Work out the finished part from the listing and answer in its coordinate system (mm). A direction names the side the tool comes from. Coordinates: 2 decimals unless noted, no trailing zeros. Order: outer loops, then holes, each group sorted by start corner. A loop starts at its lowest first (then second) coordinate and runs counter-clockwise, first axis right, second up. Notation, with made-up numbers: (-7, 13) - (40, 13) arc R23 cw to (40, 36) - close; hole circle Ø4 at (61.5, 32). An arc over 180 degrees is marked (long way). Answer as a JSON object with one key per item and string values. Group by question number.
1) Section B-B (z = -8) is taken. Give the vertices of the cut face in (x, y), plus the area to 3 significant figures.
2) Section C-C (y = -0.5) is taken. Give the vertices of the cut face in (x, z) (1 decimal).
3) Find the intervals of material crossed by line 1 along Z through (x, y) = (1.25, 0.75); line 2 along Y through (x, z) = (3.5, -3.5); line 3 along X through (y, z) = (4.75, -3.75), in increasing order.
4) A tool of negligible diameter and unlimited length cuts with its end or side. For faces 1 (the face through (-5, 0, -6)), 2 (the face through (-0.9, -0.5, 0.767)), from which of +Z, -Z, +X, -X, +Y, -Y can it reach the whole face along a straight path? Write none if from no direction.
5) Each of these flat-tipped pins is pushed along its axis until it touches: P1, Ø1.1, axis at x = 1, y = 2, coming from the +Z side; P2, Ø1.1, axis at x = -2.5, y = 2, coming from the -Z side; P3, Ø1, axis at x = -0.5, z = -4.5, coming from the +Y side. Where does it stop, or does it pass through?
6) Section A-A (y = 1.75) is taken. Give the vertices of the cut face in (x, z) (1 decimal).
Autodesk Inventor part; units mm, degrees
ref_plane "Work Plane1" through (1.3404, 0, -3.935) normal (0, 0, -1) x (-1, 0, 0)
ref_plane "YZ Plane" through (0, 0, 0) normal (1, 0, 0) x (0, 1, 0)
ref_plane "XZ Plane" through (0, 0, 0) normal (0, 1, 0) x (-1, 0, 0)
sketch "Sketch1" plane through (0, 0, 0) normal (0, 1, 0) x (-1, 0, 0)
  arc A0 (3.8736, -1.1608) -> (1.863, 0) centre (0.9315, -3.935) ccw
  line L0 (1.863, 0) -> (0, 0)
  arc A1 (0, 0) -> (-2.0106, -1.1608) centre (0.9315, -3.935) ccw
  line L1 (-2.0106, -1.1608) -> (-2.9421, -2.7742)
  arc A2 (-2.9421, -2.7742) -> (-2.9421, -5.0958) centre (0.9315, -3.935) ccw
  line L2 (-2.9421, -5.0958) -> (-2.0106, -6.7092)
  arc A3 (-2.0106, -6.7092) -> (0, -7.87) centre (0.9315, -3.935) ccw
  line L3 (0, -7.87) -> (1.863, -7.87)
  arc A4 (1.863, -7.87) -> (3.8736, -6.7092) centre (0.9315, -3.935) ccw
  line L4 (3.8736, -6.7092) -> (4.805, -5.0958)
  arc A5 (4.805, -5.0958) -> (4.805, -2.7742) centre (0.9315, -3.935) ccw
  line L5 (4.805, -2.7742) -> (3.8736, -1.1608)
  circle A6 centre (0.9315, -3.145) radius 2.5
  line L6 (-0.7685, 0.7671) -> (2.6315, 0.7671)
  arc A7 (-0.7685, 0.7671) -> (2.6315, 0.7671) centre (0.9315, -3.935) ccw
  line L7 (-1.3404, 0) -> (-3.6123, -3.935)
  line L8 (3.2034, 0) -> (-1.3404, 0)
  line L9 (5.4752, -3.935) -> (3.2034, 0)
  line L10 (3.2034, -7.87) -> (5.4752, -3.935)
  line L11 (-1.3404, -7.87) -> (3.2034, -7.87)
  line L12 (-3.6123, -3.935) -> (-1.3404, -7.87)
extrude "Extrusion1" add sketch "Sketch1" against normal blind 1 contours L5 A5 L4 A4 L3 A3 L2 A2 L1 A1 L0 A0 | A0 L8 L9 | L9 L10 A5 | A1 L7 L8 | L10 L11 A4 | A2 L12 L7 | L11 L12 A3 | L6 A7
extrude "Extrusion2" add sketch "Sketch1" along normal blind 5 contours L5 A5 L4 A4 L3 A3 L2 A2 L1 A1 L0 A0 | A0 L8 L9 | L9 L10 A5 | A1 L7 L8 | L10 L11 A4 | A2 L12 L7 | L11 L12 A3
ref_plane "Work Plane1" through (1.3404, 0, -3.935) normal (0, 0, -1) x (-1, 0, 0)
sketch "Sketch2" plane through (1.3404, 0, -3.935) normal (0, 0, -1) x (-1, 0, 0)
  line L0 (0, 5) -> (-2.2719, 5)
  line L1 (-2.2719, 0) -> (-2.2719, 5)
  line L2 (-0.2281, 5) -> (4.7719, 5)
  line L3 (0, 5) -> (4.5437, 5)
  line L4 (2.2719, 5) -> (2.2719, -2.0706)
  line L5 (-2.2719, 5) -> (0, 5)
  line L6 (-1.7719, 5) -> (-2.2719, 4.5)
  line L7 (-2.2719, 5) -> (-2.2719, 4.5)
  line L8 (-2.2719, 5) -> (-1.7719, 5)
  point P0 (1.3404, 0)
  dimension "d7" = 0.5
  dimension "d8" = 0.5
revolve "Revolution1" cut sketch "Sketch2" angle 360 about axis through (-0.9315, 5, -3.935) along (0, -1, 0)
thread "Thread1"
chamfer "Chamfer1" distance 0.2 angle 45 2 edges at (1.5685, 5, -3.145) (1.5685, -1, -3.145)
properties part number "Mini Eccentric Spacer 6mm" material "Steel"
Report:
{
 "1": {"outline": "(-3.84, -1) - (1.98, -1) - (1.98, 0) - (-3.84, 0) - close", "area": "5.82 mm²"},
 "2": {"outline": "(-2.6, 0.8) arc R5 ccw (long way) to (0.8, 0.8) - close; hole circle Ø5 at (-0.9, -3.1)"},
 "3": {"line 1": "z = -7.87 to -4.37, -1.92 to 0", "line 2": "y = -1 to 0", "line 3": "x = -5.22 to -3.36, 1.49 to 3.36"},
 "4": {"face 1": "+Y", "face 2": "+Z, +X, -X, +Y, -Y"},
 "5": {"P1": "stops at z = 0", "P2": "stops at z = -7.87", "P3": "passes through"},
 "6": {"outline": "(-5.5, -3.9) - (-4.8, -5.1) - (-3.9, -6.7) - (-3.2, -7.9) - (1.3, -7.9) - (2, -6.7) - (2.9, -5.1) - (3.6, -3.9) - (2.9, -2.8) - (2, -1.2) - (1.3, 0) - (-3.2, 0) - (-3.9, -1.2) - (-4.8, -2.8) - close; hole circle Ø5 at (-0.9, -3.1)"}
}
